Model file for the job. Use its own axes, mm. A direction names the side the tool comes from. Coordinates: 2 decimals unless noted, no trailing zeros. Order: outer loops, then holes, each group sorted by start corner. A loop starts at its lowest first (then second) coordinate and runs counter-clockwise, first axis right, second up. Notation, with made-up numbers: M -28,55.25 L -8,55.25 A33 ccw -8,91.25 Z; hole C 44.5,69.25 d4. An arc over 180 degrees is marked long. Return JSON: item names as keys, results as strings.
```python
from build123d import *

# Parameters (mm, degrees)
ESQUISSE1_W                = 150
ESQUISSE1_H                = 30
BOSS_EXTRU_1_DEPTH         = 30
BOSS_EXTRU_2_START         = -10
BOSS_EXTRU_2_DEPTH         = 20
R_P_TITION_LIN_AIRE1_COUNT = 2
R_P_TITION_LIN_AIRE1_PITCH = 75


with BuildPart() as part:
    # Esquisse1 → Boss.-Extru.1 (new body)
    with BuildSketch(Plane.XY):
        with Locations((-75, 15)):
            Rectangle(ESQUISSE1_W, ESQUISSE1_H)
    extrude(amount=BOSS_EXTRU_1_DEPTH)

    # Esquisse2 → Boss.-Extru.2 (add)
    with BuildSketch(Plane.ZY.offset(150).offset(BOSS_EXTRU_2_START)):
        Polygon((30, 27.158170339), (63.156193336, 27.158170339), (63.156193336, -24.079833233), (51.504613428, -24.079833233), (51.504613428, 13.190748461), (43.833386904, 13.190748461), (43.833386904, -24.079833233), (30, -24.079833233), align=None)
    boss_extru_2 = extrude(amount=-BOSS_EXTRU_2_DEPTH)

    # Répétition linéaire1: Boss.-Extru.2 ×2
    with Locations(*[(i * R_P_TITION_LIN_AIRE1_PITCH, 0, 0) for i in range(1, R_P_TITION_LIN_AIRE1_COUNT)]):
        add(boss_extru_2)


solid = part.part
```
Item 1: Drop flat-ended pins along their axis: pin 1 Ø5 at (x, z) = (-58, 45.5) entering from +Y; pin 2 Ø2 at (y, z) = (-11.5, 37.5) entering from +X; pin 3 Ø6 at (x, y) = (-42.5, -16) entering from -Z. Give the stop position or say it passes through.
Check result:
{"pin 1": "stops at y = 27.16", "pin 2": "stops at x = -45", "pin 3": "stops at z = 30"}
Item 2: Saw through at B-B (y = -7). Write the cut outline in (x, z).
Check result:
{"outline": "M -140,30 L -120,30 L -120,43.83 L -140,43.83 Z; M -140,51.5 L -120,51.5 L -120,63.16 L -140,63.16 Z; M -65,30 L -45,30 L -45,43.83 L -65,43.83 Z; M -65,51.5 L -45,51.5 L -45,63.16 L -65,63.16 Z"}
Item 3: Saw through at C-C (x = -131). Write the cut outline in (y, z), and give its area (3 significant figures).
Check result:
{"outline": "M -24.08,30 L 0,30 L 0,0 L 30,0 L 30,30 L 27.16,30 L 27.16,63.16 L -24.08,63.16 L -24.08,51.5 L 13.19,51.5 L 13.19,43.83 L -24.08,43.83 Z", "area": "2,310 mm2"}
Item 4: Saw through at D-D (z = 19). Write the cut outline in (x, y), and give its area (3 significant figures).
Check result:
{"outline": "M -150,0 L 0,0 L 0,30 L -150,30 Z", "area": "4,500 mm2"}
Item 5: Wall check: line 1 (X direction, y = -2, z = 57.5); line 2 (Z direction, x = -94, y = 1.5); line 3 (Y direction, x = -138.5, z = 50.5). Give the ranges that are in metal, low to high.
Check result:
{"line 1": "x = -140 to -120, -65 to -45", "line 2": "z = 0 to 30", "line 3": "y = 13.19 to 27.16"}
Item 6: Saw through at A-A (z = 57.5). Write the cut outline in (x, y).
Check result:
{"outline": "M -140,-24.08 L -120,-24.08 L -120,27.16 L -140,27.16 Z; M -65,-24.08 L -45,-24.08 L -45,27.16 L -65,27.16 Z"}
Item 7: Pull direction Z, two halves, no side cores. Call faces 1 (the flat face through (-150, 15, 15)), 2 (the flat face through (-55, -12, 30)), 3 (the flat face through (-55, -6, 51.505)), 4 (the flat face through (-130, -5, 43.833)): +Z half, -Z half, draft (parallel to the pull), parting line (faces both ways), or undercut.
Check result:
{"face 1": "draft", "face 2": "-Z half", "face 3": "undercut", "face 4": "undercut"}
Item 8: 3-axis set-ups, long thin cutter, end or side, ignore diameter. For faces 5 (the flat face through (-55, 27.158, 46)), 6 (the flat face through (-55, 2, 63.156)), 7 (the flat face through (-120, 2, 43)), 8 (the flat face through (-76, 0, 15)), 9 (the flat face through (-55, -5, 43.833)): which of +Z, -Z, +X, -X, +Y, -Y reach the whole face in a straight line?
Check result:
{"face 5": "+Z, +X, -X, +Y", "face 6": "+Z, +X, -X, +Y, -Y", "face 7": "+Z, +Y, -Y", "face 8": "-Z, +X, -X, -Y", "face 9": "+X, -X, -Y"}
